Can you work these out from the model? Positions are in its coordinate system, mm. A direction names the side the tool comes from. Give positions to 0.01 mm unless a question says otherwise; leave off trailing zeros. Write each loop counter-clockwise with the first axis right and the second up, starting at its lowest first coordinate (ties: lowest second). Pieces come first, ordered by that corner, then holes.
```python
from build123d import *

# Parameters (mm, degrees)
F1_DEPTH = 63.5
F2_DEPTH = 25.4
F3_DEPTH = 7.9375
F5_R     = 6.35


with BuildPart() as f1:
    # F0 (on Front) → F1 (new body, symmetric)
    with BuildSketch(Plane.XZ):
        Polygon((22.225, 9.525), (-41.275, 9.525), (-41.275, -9.525), (41.275, -9.525), (41.275, 9.525), align=None)
    extrude(amount=F1_DEPTH, both=True)

    # F0 (on Front) → F2 (join, symmetric)
    with BuildSketch(Plane.XZ):
        with BuildLine():
            Line((22.225, 27.147116), (22.225, 9.525))
            Line((22.225, 9.525), (41.275, 9.525))
            Line((41.275, 9.525), (41.275, 27.147116))
            ThreePointArc((41.275, 27.147116), (45.187089, 37.582842), (54.995237, 42.8752))
            Line((54.995237, 42.8752), (60.325, 42.8752))
            Line((60.325, 42.8752), (60.325, 61.9252))
            Line((60.325, 61.9252), (53.949921, 61.9252))
            ThreePointArc((53.949921, 61.9252), (31.34769, 50.684245), (22.225, 27.147116))
        make_face()
    extrude(amount=F2_DEPTH, both=True)

    # F0 (on Front) → F3 (join, symmetric)
    with BuildSketch(Plane.XZ):
        with BuildLine():
            add(Edge.make_bspline(
                [(-41.275, 9.525), (-40.190469, 45.686379), (0, 61.9252), (53.949921, 61.9252)],
                knots=[0, 0, 0, 0, 108.690232, 108.690232, 108.690232, 108.690232], degree=3))
            Line((-41.275, 9.525), (22.225, 9.525))
            Line((22.225, 9.525), (22.225, 27.147116))
            ThreePointArc((22.225, 27.147116), (31.34769, 50.684245), (53.949921, 61.9252))
        make_face()
    extrude(amount=F3_DEPTH, both=True)

    # F0 (on Front) → F4 (revolve)
    with BuildSketch(Plane.XZ):
        Polygon((60.325, 66.675), (60.325, 61.9252), (78.97443, 61.9252), (78.97443, 42.8752), (60.325, 42.8752), (60.325, 38.1), (111.125, 38.1), (111.125, 66.675), align=None)
    revolve(axis=Axis((60.325, 0, 52.3875), (0, 0, 1)))

    # F5
    f5_edges = [f1.edges().sort_by_distance(p)[0] for p in [
        (-41.275, -63.5, 0),
        (41.275, -63.5, 0),
        (41.275, 63.5, 0),
        (-41.275, 63.5, 0),
    ]]
    fillet(f5_edges, radius=F5_R)


solid = f1.part
```
1) Suppose I cut it at C-C on x = 18. Write out the boundary of the cut face in (y, z) (1 decimal).
Values follow:
outline: (-63.5, -9.5) - (63.5, -9.5) - (63.5, 9.5) - (7.9, 9.5) - (7.9, 38.1) - (28.1, 38.1) - (28.1, 66.7) - (-28.1, 66.7) - (-28.1, 38.1) - (-7.9, 38.1) - (-7.9, 9.5) - (-63.5, 9.5) - close
2) Suppose I cut it at A-A on z = 5.5. Write out the boundary of the cut face in (x, y) (3 decimals).
Values follow:
outline: (-41.275, -57.15) arc R6.35 ccw to (-34.925, -63.5) - (34.925, -63.5) arc R6.35 ccw to (41.275, -57.15) - (41.275, 57.15) arc R6.35 ccw to (34.925, 63.5) - (-34.925, 63.5) arc R6.35 ccw to (-41.275, 57.15) - close
3) Suppose I cut it at B-B on y = 32. Write out the boundary of the cut face in (x, z) (3 decimals), plus the area to 3 significant figures.
Values follow:
outline: (-41.275, -9.525) - (41.275, -9.525) - (41.275, 9.525) - (-41.275, 9.525) - close; (20.871, 38.1) - (99.779, 38.1) - (99.779, 66.675) - (20.871, 66.675) - close
area: 3,830 mm2
4) For pin 1 Ø12 at (y, z) = (-44.5, 38.5) entering from -X; pin 2 Ø24 at (x, z) = (-8, 42.5) entering from +Y; pin 3 Ø12 at (y, z) = (43, 53.5) entering from -X, each with a flat end and sliding along its axis, tell me the tip position at first contact or that it passes through.
Values follow:
pin 1: stops at x = 27.18
pin 2: stops at y = 7.94
pin 3: stops at x = 25.52
5) Please list where these lines run through material, in increasing order: L1, parallel to Y at x = -11, z = 25; L2, parallel to Z at x = 29.5, y = 40.5 (3 decimals); L3, parallel to X at y = 48, z = 6 (3 decimals).
Values follow:
L1: y = -7.94 to 7.94
L2: z = -9.525 to 9.525
L3: x = -41.275 to 41.275
6) If we mould it in two halves opening along Z, with no side actions, what happens to faces 1 (the face through (39.464, 61.59, 0.133)), 2 (the face through (60, 1, 66.675)), 3 (the face through (49.85, -11.73, 61.3))? For each: +Z half, -Z half, draft (parallel to the pull), parting line (faces both ways), or undercut.
Values follow:
face 1: draft
face 2: +Z half
face 3: undercut
7) For faces 4 (the face through (22.225, -17, 18)), 5 (the face through (-8, 7.938, 29)), 6 (the face through (107.25, -19.46, 52.59)), 7 (the face through (67, 0, 42.875)), which set-ups out of +Z, -Z, +X, -X, +Y, -Y let a thin tool reach every point of the face, with its end or its side?
Values follow:
face 4: -X, -Y
face 5: -X, +Y
face 6: +Z
face 7: none
